Could you check a few things on this drawing? It's one solid part, dimensions in mm from its lowest x, y, z. Coordinates: 2 decimals unless noted, no trailing zeros. Order: outer loops, then holes, each group sorted by start corner. A loop starts at its lowest first (then second) coordinate and runs counter-clockwise, first axis right, second up. Notation, with made-up numbers: (-20.75, 14.5) -> (30.25, 14.5) arc R17 cw to (30.25, 40.5) -> close; hole circle Ø10 at (2, 12). An arc over 180 degrees is marked (long way). Answer as CSV lines item,"result".
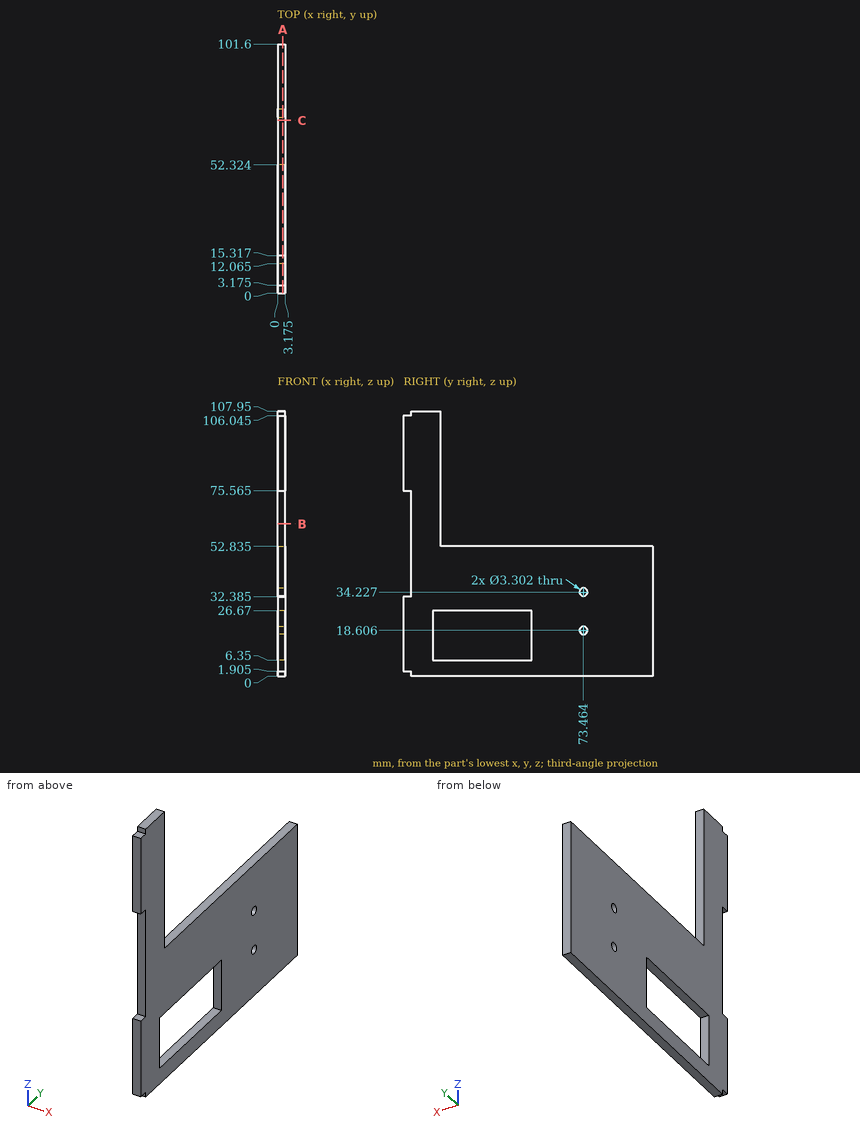
Q1. If I drill on line 1 (Z direction, x = 3, y = 74) (1 decimal); line 2 (Y direction, x = 0.25, z = 15) (1 decimal); line 3 (Z direction, x = 1.4, y = 93.5) (1 decimal), over which ranges is the centre line in solid material (lowest first)?
Solution:
line 1,"0 to 17, 20.2 to 32.7, 35.8 to 52.8"
line 2,"0 to 12.1, 52.3 to 101.6"
line 3,"0 to 52.8"
Q2. For P1, Ø1.6, axis at x = 2, y = 29.5, coming from the -Z side; P2, Ø1.6, axis at x = 2, z = 49.5, coming from the -Y side (1 decimal); P3, Ø1.6, axis at x = 1.5, z = 72, coming from the +Y side; P4, Ø1, axis at x = 1.5, y = 1, coming from the +Z side (1 decimal), each with a flat end and sliding along its axis, tell me the tip position at first contact or that it passes through.
Solution:
P1,"z = 0"
P2,"y = 3.2"
P3,"y = 15.32"
P4,"z = 106"
Q3. Imagine slicing it at C-C (y = 70.5). List the corners of the cut face in (x, z) for me (1 decimal).
Solution:
outline,"(0, 0) -> (3.2, 0) -> (3.2, 52.8) -> (0, 52.8) -> close"
Q4. Imagine slicing it at A-A (x = 2.2). Give the number of separate pieces and of enclosed holes in the cut face, and give its area (3 significant figures).
Solution:
separate pieces,"1"
enclosed holes,"3"
area,"5,230 mm2"
Q5. Imagine slicing it at B-B (z = 62). List the corners of the cut face in (x, y) for me (1 decimal).
Solution:
outline,"(0, 3.2) -> (3.2, 3.2) -> (3.2, 15.3) -> (0, 15.3) -> close"
